```python
from build123d import *

# Parameters (mm, degrees)
SKETCH_W     = 100
SKETCH_H     = 100
PAD_DEPTH    = 80
FILLET_R     = 10
THICKNESS_T  = -4
POCKET_DEPTH = 10


with BuildPart() as part:
    # Sketch → Pad (new body)
    with BuildSketch(Plane.XY):
        with Locations((50, 50)):
            Rectangle(SKETCH_W, SKETCH_H)
    extrude(amount=PAD_DEPTH)

    # Fillet
    fillet_edges = [part.edges().sort_by_distance(p)[0] for p in [
        (0, 0, 40),
        (100, 0, 40),
        (100, 100, 40),
        (0, 100, 40),
    ]]
    fillet(fillet_edges, radius=FILLET_R)

    # Thickness
    thickness_openings = [part.faces().sort_by_distance(p)[0] for p in [
        (50, 50, 80),
    ]]
    offset(amount=THICKNESS_T, openings=thickness_openings, kind=Kind.INTERSECTION)

    # Sketch001 (on Face10 of Thickness) → Pocket (cut)
    with BuildSketch(Plane.XY.offset(80)):
        with BuildLine():
            Line((0, 90), (0, 10))
            ThreePointArc((0, 10), (2.928932, 2.928932), (10, 0))
            Line((10, 0), (90, 0))
            ThreePointArc((90, 0), (97.071068, 2.928932), (100, 10))
            Line((100, 10), (100, 90))
            ThreePointArc((100, 90), (97.071068, 97.071068), (90, 100))
            Line((90, 100), (10, 100))
            ThreePointArc((10, 100), (2.928932, 97.071068), (0, 90))
        make_face()
        with BuildLine():
            Line((2, 90), (2, 10))
            ThreePointArc((2, 10), (4.343146, 4.343146), (10, 2))
            Line((10, 2), (90, 2))
            ThreePointArc((90, 2), (95.656854, 4.343146), (98, 10))
            Line((98, 10), (98, 90))
            ThreePointArc((98, 90), (95.656854, 95.656854), (90, 98))
            Line((90, 98), (10, 98))
            ThreePointArc((10, 98), (4.343146, 95.656854), (2, 90))
        make_face(mode=Mode.SUBTRACT)
    extrude(amount=-POCKET_DEPTH, mode=Mode.SUBTRACT)


solid = part.part
```
The listing builds one solid part. Answer for the finished solid, in the listing's coordinates (mm). A direction names the side the tool comes from. Give positions to 0.01 mm unless a question says otherwise; leave off trailing zeros. Order: outer loops, then holes, each group sorted by start corner. A loop starts at its lowest first (then second) coordinate and runs counter-clockwise, first axis right, second up. Notation, with made-up numbers: (-40, 16.25) -> (-23, 16.25) arc R22 ccw to (-23, 40.25) -> close; hole circle Ø2 at (-26, 43.5). An arc over 180 degrees is marked (long way). Write each question's results on one line, items separated by ' | '.
Q1. Each of these flat-tipped pins is pushed along its axis until it touches: P1, Ø8, axis at x = 47, z = 77, coming from the +Y side; P2, Ø6, axis at x = 49.5, y = 67, coming from the +Z side; P3, Ø5, axis at y = 32.5, z = 75.5, coming from the -X side. Where does it stop, or does it pass through?
Checked values:
P1: stops at y = 98 | P2: stops at z = 4 | P3: stops at x = 2
Q2. Straight lines are drawn through the part: probe 1 along X at (y, z) = (68, 24); probe 2 along X at (y, z) = (58, 70.5). For each, find the intervals that lie inside material, in ascending order. Write a range as from..to.
Checked values:
probe 1: x = 0..4, 96..100 | probe 2: x = 2..4, 96..98
Q3. Determine the mould class of faces 1 (the face through (94.196, 5.711, 42.532)), 2 (the face through (95.594, 4.281, 75.07)), 3 (the face through (4.406, 95.719, 75.07)) for opening direction Y: pulls with the +Y half, pulls with the -Y half, needs draft (parallel to the pull), parting line crosses it, or undercut.
Checked values:
face 1: undercut | face 2: pulls with the -Y half | face 3: pulls with the +Y half
Q4. The part is cut by section B-B, the plane y = 74. Give the vertices of the cut face in (x, z), and give its area (3 significant figures).
Checked values:
outline: (0, 0) -> (100, 0) -> (100, 70) -> (98, 70) -> (98, 80) -> (96, 80) -> (96, 4) -> (4, 4) -> (4, 80) -> (2, 80) -> (2, 70) -> (0, 70) -> close | area: 968 mm^2
Q5. The part is cut by section D-D, the plane z = 71.5. Give the vertices of the cut face in (x, y), and give its area (3 significant figures).
Checked values:
outline: (2, 10) arc R8 ccw to (10, 2) -> (90, 2) arc R8 ccw to (98, 10) -> (98, 90) arc R8 ccw to (90, 98) -> (10, 98) arc R8 ccw to (2, 90) -> close; hole (4, 10) arc R6 ccw to (10, 4) -> (90, 4) arc R6 ccw to (96, 10) -> (96, 90) arc R6 ccw to (90, 96) -> (10, 96) arc R6 ccw to (4, 90) -> close | area: 728 mm^2
Q6. The part is cut by section A-A, the plane z = 31. Give the vertices of the cut face in (x, y), and give its area (3 significant figures).
Checked values:
outline: (0, 10) arc R10 ccw to (10, 0) -> (90, 0) arc R10 ccw to (100, 10) -> (100, 90) arc R10 ccw to (90, 100) -> (10, 100) arc R10 ccw to (0, 90) -> close; hole (4, 10) arc R6 ccw to (10, 4) -> (90, 4) arc R6 ccw to (96, 10) -> (96, 90) arc R6 ccw to (90, 96) -> (10, 96) arc R6 ccw to (4, 90) -> close | area: 1,480 mm^2
Q7. Which of the six approach directions +Z, -Z, +X, -X, +Y, -Y give full straight-line access (tool end or side, diameter ignored) to faces 4 (the face through (49, 2, 75)), 5 (the face through (0, 49, 35)), 6 (the face through (2, 51, 75)), 7 (the face through (4, 49, 41)), 8 (the face through (51, 98, 75))?
Checked values:
face 4: +Z, +X, -X, -Y | face 5: +Z, -Z, -X, +Y, -Y | face 6: +Z, -X, +Y, -Y | face 7: +Z | face 8: +Z, +X, -X, +Y
